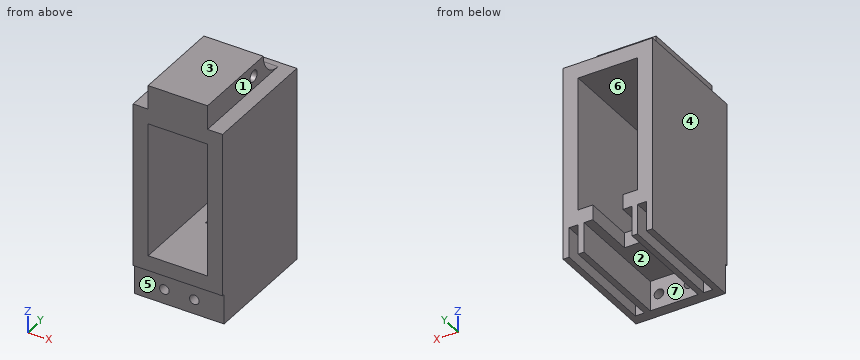
from build123d import *

# Parameters (mm, degrees)
BOSS_EXTRUDE1_DEPTH     = 50.8
CUT_EXTRUDE1_DEPTH      = 92.455090356
CUT_EXTRUDE1_DEPTH_BACK = 50.8
SKETCH4_W               = 37.846
SKETCH4_H               = 12.7
SKETCH4_R               = 2.032
BOSS_EXTRUDE2_DEPTH     = 4.572
SKETCH7_W               = 2.54
SKETCH7_H               = 12.7
SKETCH7_W_2             = 2.353491512
BOSS_EXTRUDE3_DEPTH     = 45.212
BOSS_EXTRUDE4_DEPTH     = 37.846
FILLET1_R               = 10.16
SKETCH9_W               = 6.35
SKETCH9_H               = 13.184190116
CUT_EXTRUDE2_DEPTH      = 94.73231429


with BuildPart() as part:
    # Sketch1 → Boss-Extrude1 (new body)
    with BuildSketch(Plane(origin=(0, 0, 0), x_dir=(1, 0, 0), z_dir=(0, 1, 0))):
        Polygon((-24.306, -56.0525), (-24.306, -27.6045), (-30.656, -27.6045), (-30.656, -62.4025), (7.19, -62.4025), (7.19, 7.1935), (-11.733, 7.1935), (-11.733, 0.8435), (0.84, 0.8435), (0.84, -56.0525), align=None)
        Polygon((-24.306, -27.6045), (-24.306, 0.8435), (-11.733, 0.8435), (-11.733, 7.1935), (-30.656, 7.1935), (-30.656, -27.6045), align=None)
    extrude(amount=BOSS_EXTRUDE1_DEPTH)

    # Sketch3 → Cut-Extrude1 (cut, two sides: drawn at the far end of the back side and taken through both)
    with BuildSketch(Plane(origin=(0, 0, -7.1935), x_dir=(-1, 0, 0), z_dir=(0, 0, -1)).offset(-CUT_EXTRUDE1_DEPTH_BACK)):
        Polygon((5.383, 29.21), (11.733, 29.21), (18.083, 29.21), (18.083, 50.8), (5.383, 50.8), align=None)
    extrude(amount=CUT_EXTRUDE1_DEPTH + CUT_EXTRUDE1_DEPTH_BACK, mode=Mode.SUBTRACT)

    # Sketch4 → Boss-Extrude2 (add)
    with BuildSketch(Plane(origin=(0, 1.016, 0), x_dir=(1, 0, 0), z_dir=(0, 1, 0))):
        with Locations((-11.733, 13.5435)):
            Rectangle(SKETCH4_W, SKETCH4_H)
        with Locations(Location((-18.083, 13.7975, 0), (0, 0, 270))):
            Circle(SKETCH4_R, mode=Mode.SUBTRACT)
        with Locations(Location((-5.383, 13.7975, 0), (0, 0, 270))):
            Circle(SKETCH4_R, mode=Mode.SUBTRACT)
    extrude(amount=BOSS_EXTRUDE2_DEPTH)

    # Sketch7 → Boss-Extrude3 (add)
    with BuildSketch(Plane(origin=(0, 5.588, 0), x_dir=(1, 0, 0), z_dir=(0, 1, 0))):
        with Locations((5.92, 13.5435)):
            Rectangle(SKETCH7_W, SKETCH7_H)
        with Locations((-0.43, 13.5435)):
            Rectangle(SKETCH7_W, SKETCH7_H)
        with Locations((-23.129254244, 13.5435)):
            Rectangle(SKETCH7_W_2, SKETCH7_H)
        with Locations((-29.386, 13.5435)):
            Rectangle(SKETCH7_W, SKETCH7_H)
    extrude(amount=BOSS_EXTRUDE3_DEPTH)

    # Sketch8 → Boss-Extrude4 (add)
    with BuildSketch(Plane.ZY.offset(30.656)):
        with BuildLine():
            Line((71.5465, 31.496), (70.1495, 31.496))
            ThreePointArc((70.1495, 31.496), (67.7365, 29.083), (65.3235, 31.496))
            Line((65.3235, 31.496), (62.4025, 31.496))
            Line((62.4025, 31.496), (62.4025, 0))
            Line((62.4025, 0), (71.5465, 0))
            Line((71.5465, 0), (71.5465, 31.496))
        make_face()
        with BuildLine():
            ThreePointArc((65.3235, 31.496), (67.7365, 33.909), (70.1495, 31.496))
            Line((70.1495, 31.496), (71.5465, 31.496))
            Line((71.5465, 31.496), (71.5465, 0))
            Line((71.5465, 0), (72.5625, 0))
            Line((72.5625, 0), (72.5625, 38.1))
            Line((72.5625, 38.1), (62.4025, 38.1))
            Line((62.4025, 38.1), (62.4025, 31.496))
            Line((62.4025, 31.496), (65.3235, 31.496))
        make_face()
    extrude(amount=-BOSS_EXTRUDE4_DEPTH)

    # Fillet1
    fillet1_edges = [part.edges().sort_by_distance(p)[0] for p in [
        (-11.733, 38.1, 62.4025),
    ]]
    fillet(fillet1_edges, radius=FILLET1_R - 0.0001)  # a hair under: the kernel refuses the full size

    # Sketch9 → Cut-Extrude2 (cut, through all)
    with BuildSketch(Plane(origin=(0, 50.8, 0), x_dir=(1, 0, 0), z_dir=(0, 1, 0))):
        with Locations((-27.481, -68.994595058)):
            Rectangle(SKETCH9_W, SKETCH9_H)
        Polygon((7.19, -62.4025), (0.84, -62.4025), (0.84, -76.255559197), (7.295762748, -76.255559197), align=None)
    extrude(amount=-CUT_EXTRUDE2_DEPTH, mode=Mode.SUBTRACT)


solid = part.part
Input: part model. Units: mm. Frame: model coordinates. Face numbers are marked on the shaded views. A direction names the side the tool comes from. Give positions to 0.01 mm unless a question says otherwise; leave off trailing zeros. Loops run counter-clockwise (first coordinate to the right, second up) from the corner with the lowest first, then second, coordinate; pieces in that order, holes last. Notation, with made-up numbers: (67.5, -3) -> (88.5, -3) arc R4 cw to (88.5, 3) -> close; hole circle Ø8 at (-5.5, 68). An arc over 180 degrees is marked (long way). Answer as a JSON object with one key per item and string values. Group by question number.
Item 1: Line query: probe 1 along X at (y, z) = (19.5, -12.5); probe 2 along X at (y, z) = (35, 3.5); probe 3 along Z at (x, y) = (-5, 28.5). Output: solid intervals per line, ascending.
Item 2: Reachability of the marked faces 5, 6 and 7 from +Z, -Z, +X, -X, +Y, -Y: full face, straight path, thin tool, end or side. Return the list, or none.
Item 3: Pin query (flat end, axial travel): P1, Ø3, axis at y = 31.5, z = 67.74, coming from the +X side; P2, Ø1.9, axis at x = -14.5, z = -3.5, coming from the +Y side; P3, Ø11, axis at y = 15, z = 69.5, coming from the -X side; P4, Ø1.9, axis at x = -26.5, z = -11.5, coming from the +Y side. Return the tip coordinate at first contact, or that it passes through.
Item 4: Cut plane A-A, the plane z = 53. Return the cut outline in (x, y), and give its area (3 significant figures).
Item 5: Cut plane D-D, the plane x = 2. Return the cut outline in (y, z).
Item 6: Cut plane C-C, the plane y = 19.5. Return the cut outline in (x, z).
Item 7: Pull-direction query (X, two-part tool) for the marked faces 1, 2, 3 and 4; classes: released by +X, released by -X, zero draft, split by the parting line, or undercut.
Item 8: Cut plane B-B, the plane x = -10.5. State how many separate pieces and enclosed holes the cut face has, and give its area (3 significant figures).
Checks:
{
 "1": {"probe 1": "x = -30.66 to -28.12, -24.31 to -21.95, -1.7 to 0.84, 4.65 to 7.19", "probe 2": "x = -30.66 to -24.31, 0.84 to 7.19", "probe 3": "z = -7.19 to -0.84, 56.05 to 72.56"},
 "2": {"face 5": "-Z, +X, -X, -Y", "face 6": "+Y, -Y", "face 7": "-Z, +Y"},
 "3": {"P1": "passes through", "P2": "stops at y = 29.21", "P3": "stops at x = -24.31", "P4": "stops at y = 5.59"},
 "4": {"outline": "(-30.66, 0) -> (-24.31, 0) -> (-24.31, 50.8) -> (-30.66, 50.8) -> close; (0.84, 0) -> (7.19, 0) -> (7.19, 50.8) -> (0.84, 50.8) -> close", "area": "645 mm²"},
 "5": {"outline": "(0, -7.19) -> (1.02, -7.19) -> (1.02, -19.89) -> (5.59, -19.89) -> (5.59, -7.19) -> (50.8, -7.19) -> (50.8, 62.4) -> (0, 62.4) -> close"},
 "6": {"outline": "(-30.66, -19.89) -> (-28.12, -19.89) -> (-28.12, -7.19) -> (-24.31, -7.19) -> (-24.31, -19.89) -> (-21.95, -19.89) -> (-21.95, -7.19) -> (-1.7, -7.19) -> (-1.7, -19.89) -> (0.84, -19.89) -> (0.84, -7.19) -> (4.65, -7.19) -> (4.65, -19.89) -> (7.19, -19.89) -> (7.19, 62.4) -> (0.84, 62.4) -> (0.84, 72.56) -> (-24.31, 72.56) -> (-24.31, 62.4) -> (-30.66, 62.4) -> close; hole (-24.31, -0.84) -> (0.84, -0.84) -> (0.84, 56.05) -> (-24.31, 56.05) -> close"},
 "7": {"face 1": "released by +X", "face 2": "undercut", "face 3": "zero draft", "face 4": "released by -X"},
 "8": {"separate pieces": "2", "enclosed holes": "1", "area": "957 mm²"}
}
